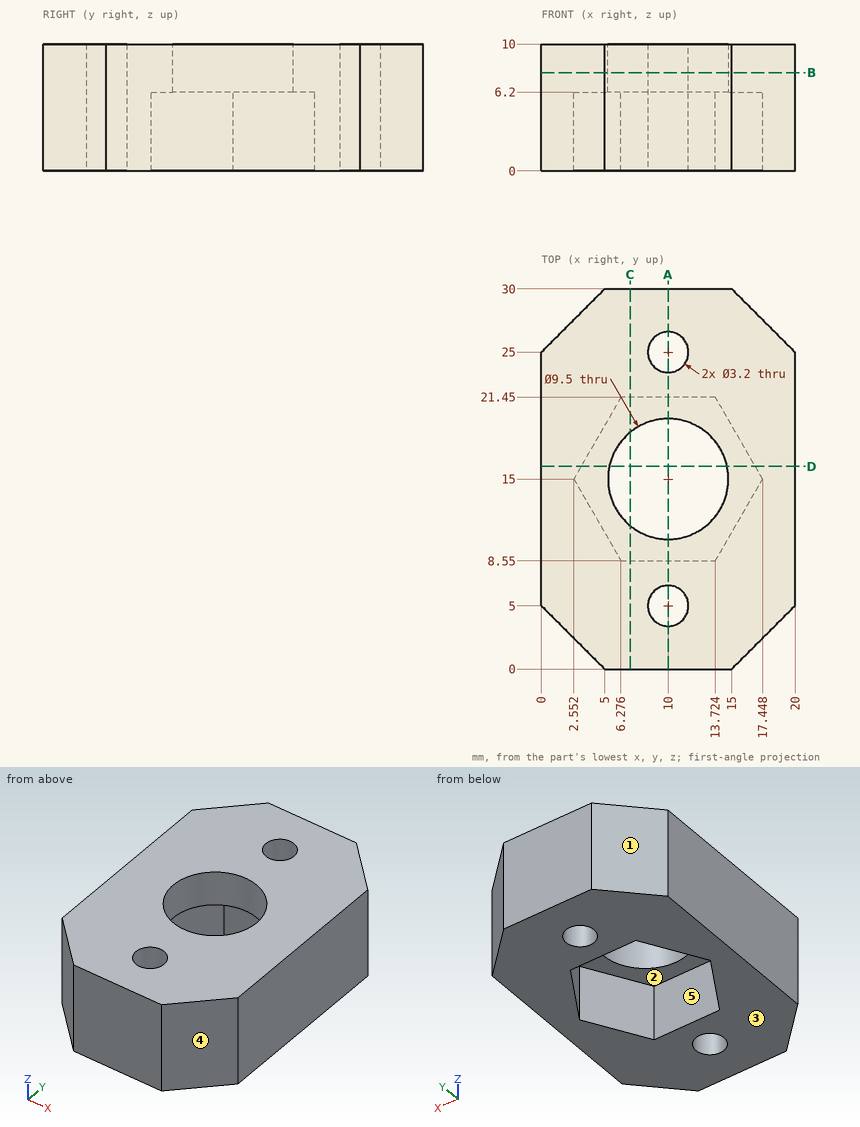
Here's the drawing with two shaded views (mm, measured from the low corner). I have some questions. A direction names the side the tool comes from. Round coordinates to 2 decimals unless told otherwise and drop trailing zeros. Write each loop counter-clockwise with the first axis right and the second up, starting at its lowest first coordinate (ties: lowest second). Pieces come first, ordered by that corner, then holes. Notation, with made-up numbers: M 75,25 L 116,25 A6 ccw 116,36 Z; hole C 89,-3 d6. An arc over 180 degrees is marked long. Answer in a Markdown table with one row per item. Add a question column.
Q1. Imagine slicing it at D-D (y = 16). Please give me the cut outline in (x, z).
Q2. Will these pins go through, and if not, where does the flat tip stop? pin 1 Ø11 at (x, y) = (10, 15) entering from +Z; pin 2 Ø4 at (x, y) = (14, 16) entering from -Z.
Q3. Imagine slicing it at B-B (z = 7.75). Please give me the cut outline in (x, y).
Q4. On a 3-axis mill with a long thin cutter (end or side, diameter ignored), from which of +Z, -Z, +X, -X, +Y, -Y can I reach the whole of each face in a straight line? I mean the marked faces 4 and 5. Say none if no direction works.
Q5. If we mould it in two halves opening along Y, with no side actions, what happens to the marked faces 1, 2 and 3? For each: +Y half, -Y half, draft (parallel to the pull), parting line (faces both ways), or undercut.
Q6. Imagine slicing it at C-C (x = 7). Please give me the cut outline in (y, z), then the cut area to 3 significant figures.
Q7. Imagine slicing it at A-A (x = 10). Please give me the cut outline in (y, z).
Q8. If I drill on line 1 (Y direction, x = 10, z = 4); line 2 (Y direction, x = 10, z = 8); line 3 (Z direction, x = 14.75, y = 11.25), over which ranges is the centre line in solid material (lowest first)? Write a range as from..to.
Values:
| question | item | result |
|---|---|---|
| 1 | outline | M 0,0 L 3.13,0 L 3.13,6.2 L 5.36,6.2 L 5.36,10 L 0,10 Z; M 14.64,6.2 L 16.87,6.2 L 16.87,0 L 20,0 L 20,10 L 14.64,10 Z |
| 2 | pin 1 | z = 10 |
| 2 | pin 2 | z = 6.2 |
| 3 | outline | M 0,5 L 5,0 L 15,0 L 20,5 L 20,25 L 15,30 L 5,30 L 0,25 Z; hole C 10,15 d9.5; hole C 10,5 d3.2; hole C 10,25 d3.2 |
| 4 | face 4 | +Z, -Z, +X, -Y |
| 4 | face 5 | -Z |
| 5 | face 1 | +Y half |
| 5 | face 2 | undercut |
| 5 | face 3 | draft |
| 6 | outline | M 0,0 L 8.55,0 L 8.55,6.2 L 11.32,6.2 L 11.32,10 L 0,10 Z; M 18.68,6.2 L 21.45,6.2 L 21.45,0 L 30,0 L 30,10 L 18.68,10 Z |
| 6 | area | 192 mm^2 |
| 7 | outline | M 0,0 L 3.4,0 L 3.4,10 L 0,10 Z; M 6.6,0 L 8.55,0 L 8.55,6.2 L 10.25,6.2 L 10.25,10 L 6.6,10 Z; M 19.75,6.2 L 21.45,6.2 L 21.45,0 L 23.4,0 L 23.4,10 L 19.75,10 Z; M 26.6,0 L 30,0 L 30,10 L 26.6,10 Z |
| 8 | line 1 | 0..3.4, 6.6..8.55, 21.45..23.4, 26.6..30 |
| 8 | line 2 | 0..3.4, 6.6..10.25, 19.75..23.4, 26.6..30 |
| 8 | line 3 | 6.2..10 |
